Autodesk Fusion 360 part; units mm, degrees
sketch "Sketch1" plane through (0, 0, 0) normal (0, 0, 1) x (1, 0, 0)
  line L0 (0, 0) -> (135, 0)
  line L1 (135, 0) -> (135, 40)
  line L2 (135, 40) -> (0, 40)
  line L3 (0, 40) -> (0, 0)
  line L4 (3.5, 36.5) -> (132.5, 36.5)
  line L5 (132.5, 36.5) -> (132.5, 3.5)
  line L6 (132.5, 3.5) -> (3.5, 3.5)
  line L7 (3.5, 3.5) -> (3.5, 36.5)
  dimension "d1" = 135
  dimension "d2" = 129
  dimension "d3" = 33
  dimension "d4" = 40
  dimension "d5" = 3.5
  dimension "d6" = 3.5
extrude "Extrude2" add sketch "Sketch1" along normal blind 14
fillet "Fillet2" radius 3 4 edges at (135, 0, 7) (135, 40, 7) (0, 0, 7) (0, 40, 7)
extrude "Extrude1" [suppressed]
fillet "Fillet1" [suppressed]
Input: part model. Units: mm. Frame: model coordinates. A direction names the side the tool comes from. Coordinates: 2 decimals unless noted, no trailing zeros. Order: outer loops, then holes, each group sorted by start corner. A loop starts at its lowest first (then second) coordinate and runs counter-clockwise, first axis right, second up. Notation, with made-up numbers: M 58.5,-16.75 L 87.5,-16.75 A34 cw 87.5,13.25 Z; hole C 29,62 d10. An arc over 180 degrees is marked long. Answer as CSV lines item,"result".
1. Pull-direction query (X, two-part tool) for faces 1 (the flat face through (69, 3.5, 7)), 2 (the cylindrical face through (0.9, 39.14, 7.1)), 3 (the flat face through (57, 2, 0)); classes: released by +X, released by -X, zero draft, split by the parting line, or undercut.
Reported:
face 1,"undercut"
face 2,"released by -X"
face 3,"zero draft"
2. Access query for faces 4 (the flat face through (0, 20, 7)), 5 (the flat face through (67, 36.5, 7)). Directions: +Z, -Z, +X, -X, +Y, -Y. A direction counts if a zero-diameter tool reaches every point of the face in a straight line with its end or side. Return the directions, or none.
Reported:
face 4,"+Z, -Z, -X, +Y, -Y"
face 5,"+Z, -Z"
3. Material intervals for line 1 (Y direction, x = 83.5, z = 6); line 2 (X direction, y = 13, z = 5), sorted ascending. Write a range as from..to.
Reported:
line 1,"0..3.5, 36.5..40"
line 2,"0..3.5, 132.5..135"
4. Section B-B (y = 22). Return the cut outline in (x, z).
Reported:
outline,"M 0,0 L 3.5,0 L 3.5,14 L 0,14 Z; M 132.5,0 L 135,0 L 135,14 L 132.5,14 Z"
5. Section A-A (x = 115). Return the cut outline in (y, z), then the cut area to 3 significant figures.
Reported:
outline,"M 0,0 L 3.5,0 L 3.5,14 L 0,14 Z; M 36.5,0 L 40,0 L 40,14 L 36.5,14 Z"
area,"98.0 mm2"
6. Section C-C (z = 7.25). Return the cut outline in (x, y), then the cut area to 3 significant figures.
Reported:
outline,"M 0,3 A3 ccw 3,0 L 132,0 A3 ccw 135,3 L 135,37 A3 ccw 132,40 L 3,40 A3 ccw 0,37 Z; hole M 3.5,3.5 L 132.5,3.5 L 132.5,36.5 L 3.5,36.5 Z"
area,"1,140 mm2"
